Here's how the part is built. I have some questions about the finished solid (model axes, mm). Face numbers are marked on the shaded views. A direction names the side the tool comes from. Coordinates: 2 decimals unless noted, no trailing zeros. Write each loop counter-clockwise with the first axis right and the second up, starting at its lowest first coordinate (ties: lowest second). Pieces come first, ordered by that corner, then holes. Notation, with made-up numbers: (-7, 60.25) -> (6, 60.25) arc R7 ccw to (6, 67.25) -> close; hole circle Ø2 at (20, -24). An arc over 180 degrees is marked (long way). Use a Markdown table: item, result. Add a question column.
Item 1: Imagine slicing it at A-A, the plane z = 0. Write out the boundary of the cut face in (x, y).
Item 2: Will these pins go through, and if not, where does the flat tip stop? pin 1 Ø0.6 at (x, y) = (11.5, 1) entering from +Z; pin 2 Ø0.6 at (x, z) = (12, -1) entering from +Y; pin 3 Ø0.9 at (x, z) = (12, 0) entering from +Y; pin 4 Ø1 at (x, y) = (9, 2) entering from +Z.
Item 3: On a 3-axis mill with a long thin cutter (end or side, diameter ignored), from which of +Z, -Z, +X, -X, +Y, -Y can I reach the whole of each face in a straight line? I mean the marked faces 4, 5 and 6. Say none if no direction works.
Item 4: If I drill on line 1 along X through (y, z) = (2.5, 1.25); line 2 along X through (y, z) = (0.75, 1); line 3 along Z through (x, y) = (11, -0.5), over which ranges is the centre line in solid material (lowest first)? Write a range as from..to.
Item 5: Imagine slicing it at C-C, the plane x = 8. Write out the boundary of the cut face in (y, z), and give its area (3 significant figures).
Item 6: If we mould it in two halves opening along Y, with no side actions, what happens to the marked faces 1, 2 and 3? For each: pulls with the +Y half, pulls with the -Y half, needs draft (parallel to the pull), parting line crosses it, or undercut.
Item 7: Imagine slicing it at D-D, the plane x = 2.75. Write out the boundary of the cut face in (y, z).
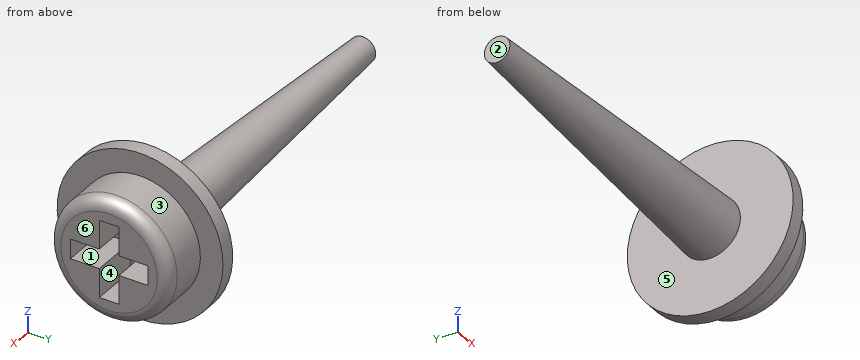
```python
from build123d import *

# Parameters (mm, degrees)
ESQUISSE5_R             = 3.3
BOSS_EXTRU_3_DEPTH      = 0.6
ESQUISSE6_R             = 2.4
BOSS_EXTRU_4_DEPTH      = 1.92
ENL_V_MAT_EXTRU_2_DEPTH = 1.92
CONG_2_R                = 0.36
CONG_3_R                = 0.48


with BuildPart() as part:
    # Esquisse4 → Révolution2 (revolve)
    with BuildSketch(Plane.XY, mode=Mode.PRIVATE) as r_volution2_sk:
        Polygon((10.181803279, 0), (-3.018196721, 0), (-3.018196721, -0.51), (10.181803279, -1.2), align=None)
    revolve(r_volution2_sk.sketch.rotate(Axis((-3.018196721, 0, 0), (1, 0, 0)), 270), axis=Axis((-3.018196721, 0, 0), (1, 0, 0)))

    # Esquisse5 → Boss.-Extru.3 (add)
    with BuildSketch(Plane(origin=(10.181803279, 0, 0), x_dir=(0, 0, -1), z_dir=(1, 0, 0))):
        Circle(ESQUISSE5_R)
    extrude(amount=BOSS_EXTRU_3_DEPTH)

    # Esquisse6 → Boss.-Extru.4 (add)
    with BuildSketch(Plane(origin=(10.781803279, 0, 0), x_dir=(0, 0, -1), z_dir=(1, 0, 0))):
        Circle(ESQUISSE6_R)
    extrude(amount=BOSS_EXTRU_4_DEPTH)

    # Esquisse7 → Enlèv. mat.-Extru.2 (cut)
    with BuildSketch(Plane(origin=(12.701803279, 0, 0), x_dir=(0, 0, -1), z_dir=(1, 0, 0))):
        Polygon((-0.39, 1.54), (0.39, 1.54), (0.39, 0.39), (1.536, 0.39), (1.536, -0.39), (0.39, -0.39), (0.39, -1.54), (-0.39, -1.54), (-0.39, -0.39), (-1.536, -0.39), (-1.536, 0.39), (-0.39, 0.39), align=None)
    extrude(amount=-ENL_V_MAT_EXTRU_2_DEPTH, mode=Mode.SUBTRACT)

    # Congé2
    cong_2_edges = [part.edges().sort_by_distance(p)[0] for p in [
        (10.781803279, -1.54, 0),
        (10.781803279, 0, 1.536),
        (10.781803279, 1.54, 0),
        (10.781803279, 0, -1.536),
    ]]
    fillet(cong_2_edges, radius=CONG_2_R)

    # Congé3
    cong_3_edges = [part.edges().sort_by_distance(p)[0] for p in [
        (12.701803279, 0, 2.4),
    ]]
    fillet(cong_3_edges, radius=CONG_3_R)


solid = part.part
```
Ans:
| question | item | result |
|---|---|---|
| 1 | outline | (-3.02, -0.51) -> (10.18, -1.2) -> (10.18, -3.3) -> (10.78, -3.3) -> (10.78, -2.4) -> (12.22, -2.4) arc R0.48 ccw to (12.7, -1.92) -> (12.7, -1.54) -> (11.14, -1.54) arc R0.36 cw to (10.78, -1.18) -> (10.78, 1.18) arc R0.36 cw to (11.14, 1.54) -> (12.7, 1.54) -> (12.7, 1.92) arc R0.48 ccw to (12.22, 2.4) -> (10.78, 2.4) -> (10.78, 3.3) -> (10.18, 3.3) -> (10.18, 1.2) -> (-3.02, 0.51) -> close |
| 2 | pin 1 | stops at z = 2.3 |
| 2 | pin 2 | stops at y = 2.3 |
| 2 | pin 3 | stops at y = 2.4 |
| 2 | pin 4 | passes through |
| 3 | face 4 | +X |
| 3 | face 5 | -X |
| 3 | face 6 | +Z, -Z, +X, +Y, -Y |
| 4 | line 1 | x = 10.18..10.78 |
| 4 | line 2 | x = 10.18..12.7 |
| 4 | line 3 | z = -2.35..-0.39, 0.39..2.35 |
| 5 | outline | circle Ø2.17 at (0, 0) |
| 5 | area | 3.70 mm^2 |
| 6 | face 1 | undercut |
| 6 | face 2 | needs draft |
| 6 | face 3 | parting line crosses it |
| 7 | outline | circle Ø1.62 at (0, 0) |
